Check sheet for the modelled part. Datum: model origin and axes. Units: mm. Face numbers are marked on the shaded views. A direction names the side the tool comes from. Give positions to 0.01 mm unless a question says otherwise; leave off trailing zeros. Loops run counter-clockwise (first coordinate to the right, second up) from the corner with the lowest first, then second, coordinate; pieces in that order, holes last. Notation, with made-up numbers: M 6.25,86 L 10.25,86 A26 cw 10.25,114 Z; hole C 55,-26.75 d8. An arc over 180 degrees is marked long. Write each question's results on one line, items separated by ' | '. Start each with the question number.
1. Sectioned sample at C-C on y = 18. Record the cut outline in (x, z) (3 decimals).
2. Sectioned sample at A-A on y = -13. Record the cut outline in (x, z) (3 decimals), and give its area (3 significant figures).
3. Draft check along Z on the marked faces 4, 5 and 6. Enter one of: pulls with the +Z half, pulls with the -Z half, needs draft (parallel to the pull), parting line crosses it, or undercut.
4. Sectioned sample at D-D on z = 59.69. Record the cut outline in (x, y) (3 decimals), and give its area (3 significant figures).
5. Go/stop test with flat-tipped pins: pin 1 (19 mm diameter, centred on x = 6, y = -13.5, fed in from +Z); pin 2 (10 mm diameter, centred on y = -3.5, z = 7.5, fed in from +X) (3 decimals); pin 3 (4.5 mm diameter, centred on y = -14, z = 16.5, fed in from -X) (3 decimals). Record where each tip stops, or that it passes through.
6. Tool access check on the marked faces 1, 2 and 3. Record the directions out of +Z, -Z, +X, -X, +Y, -Y that give a thin tool (end or side, any length) a straight path to the whole face; none if there is none.
7. Sectioned sample at B-B on x = 48. Record the cut outline in (y, z) (3 decimals), and give its area (3 significant figures).
8. Material ranges on line 1 along Z through (x, y) = (51, 18.5); line 2 along Y through (x, z) = (63.5, 81.75) (3 decimals); line 3 along Y through (x, z) = (122, 36) (3 decimals), recorded low to high.
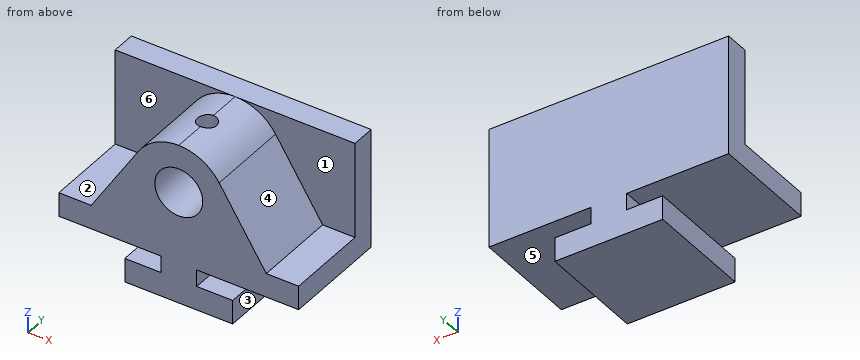
```python
from build123d import *

# Parameters (mm, degrees)
F0_W     = 127
F0_H     = 85.09
F1_DEPTH = 28.575
F3_DEPTH = 57.151
F5_R     = 5.08
F6_DEPTH = 25.4
F4_R     = 12.7
F7_DEPTH = 44.45


with BuildPart() as f1:
    # F0 (on Front) → F1 (new body, symmetric)
    with BuildSketch(Plane.XZ):
        with Locations((63.5, 42.545)):
            Rectangle(F0_W, F0_H)
    extrude(amount=F1_DEPTH, both=True)

    # F2 (on face) → F3 (cut, through all)
    with BuildSketch(Plane.XZ.offset(28.575)):
        Polygon((0, 0), (34.925, 0), (34.925, 12.7), (53.975, 12.7), (53.975, 21.59), (0, 21.59), align=None)
        Polygon((92.075, 12.7), (92.075, 0), (127, 0), (127, 21.59), (73.025, 21.59), (73.025, 12.7), align=None)
    extrude(amount=-F3_DEPTH, mode=Mode.SUBTRACT)

    # F5 (on face) → F6 (cut)
    with BuildSketch(Plane.XY.offset(85.09)):
        with Locations((63.5, -6.35)):
            Circle(F5_R)
    extrude(amount=-F6_DEPTH, mode=Mode.SUBTRACT)

    # F4 (on face) → F7 (cut)
    with BuildSketch(Plane.XZ.offset(28.575)):
        with Locations((63.5, 59.69)):
            Circle(F4_R)
        with BuildLine():
            Line((0, 85.09), (0, 34.29))
            Line((0, 34.29), (17.145, 34.29))
            Line((17.145, 34.29), (42.092005, 73.359592))
            ThreePointArc((42.092005, 73.359592), (51.29442, 81.965184), (63.5, 85.09))
            Line((63.5, 85.09), (0, 85.09))
        make_face()
        with BuildLine():
            Line((127, 85.09), (63.5, 85.09))
            ThreePointArc((63.5, 85.09), (75.70558, 81.965184), (84.907995, 73.359592))
            Line((84.907995, 73.359592), (109.855, 34.29))
            Line((109.855, 34.29), (127, 34.29))
            Line((127, 34.29), (127, 85.09))
        make_face()
    extrude(amount=-F7_DEPTH, mode=Mode.SUBTRACT)


solid = f1.part
```
Output values:
1) outline: M 0,21.59 L 53.975,21.59 L 53.975,12.7 L 34.925,12.7 L 34.925,0 L 92.075,0 L 92.075,12.7 L 73.025,12.7 L 73.025,21.59 L 127,21.59 L 127,85.09 L 0,85.09 Z
2) outline: M 0,21.59 L 53.975,21.59 L 53.975,12.7 L 34.925,12.7 L 34.925,0 L 92.075,0 L 92.075,12.7 L 73.025,12.7 L 73.025,21.59 L 127,21.59 L 127,34.29 L 109.855,34.29 L 84.908,73.36 A25.4 ccw 63.5,85.09 A25.4 ccw 42.092,73.36 L 17.145,34.29 L 0,34.29 Z; hole C 63.5,59.69 d25.4 | area: 5,000 mm2
3) face 4: pulls with the +Z half | face 5: undercut | face 6: needs draft
4) outline: M 0,15.875 L 33.364,15.875 L 33.364,-28.575 L 50.8,-28.575 L 50.8,15.875 L 76.2,15.875 L 76.2,-28.575 L 93.636,-28.575 L 93.636,15.875 L 127,15.875 L 127,28.575 L 0,28.575 Z | area: 3,160 mm2
5) pin 1: z = 34.29 | pin 2: x = 92.075 | pin 3: x = 53.975
6) face 1: +Z, +X, -Y | face 2: +Z, -X, -Y | face 3: -Z, +X, +Y, -Y
7) outline: M -28.575,0 L 28.575,0 L 28.575,12.7 L -28.575,12.7 Z; M -28.575,21.59 L 28.575,21.59 L 28.575,85.09 L 15.875,85.09 L 15.875,79.812 L -28.575,79.812 Z | area: 4,120 mm2
8) line 1: 0 to 12.7, 21.59 to 85.09 | line 2: -28.575 to -11.43, -1.27 to 28.575 | line 3: 15.875 to 28.575
